Check sheet for the modelled part. Datum: model origin and axes. Units: mm. A direction names the side the tool comes from. Round coordinates to 2 decimals unless told otherwise and drop trailing zeros. Write each loop counter-clockwise with the first axis right and the second up, starting at its lowest first coordinate (ties: lowest second). Pieces come first, ordered by that corner, then holes.
Item 1: Release check for a two-part mould opening along Y. For faces 3 (the cylindrical face through (6.691, -12.864, -2.535)), 4 (the cylindrical face through (-17.34, -78.1, -0.07)), 5 (the flat face through (17, 1, 5)) record: +Y half, -Y half, draft (parallel to the pull), parting line (faces both ways), or undercut.
Item 2: Go/stop test with flat-tipped pins: pin 1 Ø5 at (y, z) = (-33, 1) entering from +X; pin 2 Ø1 at (x, z) = (-13, 3) entering from -Y; pin 3 Ø2 at (x, z) = (7, 0) entering from -Y. Record where each tip stops, or that it passes through.
Item 3: Material ranges on line 1 (Y direction, x = 0, z = -2.9); line 2 (Y direction, x = -6, z = -4); line 3 (Z direction, x = -16, y = -27.5), recorded low to high.
Item 4: Cross-section at D-D on x = 39.5. Enter the section's corners in (y, z), plus the area to 3 significant figures.
Item 5: Cross-section at A-A on y = 0. Enter the section's corners in (x, z).
Item 6: Cross-section at C-C on z = 2. Enter the section's corners in (x, y), plus the area to 3 significant figures.
Item 7: Tool access check on faces 1 (the flat face through (2, 12, -5)), 2 (the cylindrical face through (-58.23, 53.39, -2.54)). Record the directions out of +Z, -Z, +X, -X, +Y, -Y that give a thin tool (end or side, any length) a straight path to the whole face; none if there is none.
from build123d import *

# Parameters (mm, degrees)
SKETCH1_R           = 80
SKETCH1_R_2         = 12
BOSS_EXTRUDE1_DEPTH = 5
BOSS_EXTRUDE2_START = -10
SKETCH2_R           = 14.5
SKETCH2_R_2         = 12
BOSS_EXTRUDE2_DEPTH = 10
BOSS_EXTRUDE3_START = -10
SKETCH3_R           = 80
SKETCH3_R_2         = 79
BOSS_EXTRUDE3_DEPTH = 10


with BuildPart() as part:
    # Sketch1 → Boss-Extrude1 (new body)
    with BuildSketch(Plane.XY):
        Circle(SKETCH1_R)
        Circle(SKETCH1_R_2, mode=Mode.SUBTRACT)
    extrude(amount=BOSS_EXTRUDE1_DEPTH)

    # Sketch2 → Boss-Extrude2 (add)
    with BuildSketch(Plane.XY.offset(5).offset(BOSS_EXTRUDE2_START)):
        Circle(SKETCH2_R)
        Circle(SKETCH2_R_2, mode=Mode.SUBTRACT)
    extrude(amount=BOSS_EXTRUDE2_DEPTH)

    # Sketch3 → Boss-Extrude3 (add)
    with BuildSketch(Plane.XY.offset(5).offset(BOSS_EXTRUDE3_START)):
        Circle(SKETCH3_R)
        Circle(SKETCH3_R_2, mode=Mode.SUBTRACT)
    extrude(amount=BOSS_EXTRUDE3_DEPTH)


solid = part.part
Response values:
1. face 3: undercut
1. face 4: parting line
1. face 5: draft
2. pin 1: stops at x = 73.96
2. pin 2: stops at y = -79.02
2. pin 3: stops at y = -79.77
3. line 1: y = -80 to -79, -14.5 to -12, 12 to 14.5, 79 to 80
3. line 2: y = -79.77 to -78.77, -13.2 to -10.39, 10.39 to 13.2, 78.77 to 79.77
3. line 3: z = 0 to 5
4. outline: (-69.57, -5) - (-68.42, -5) - (-68.42, 0) - (68.42, 0) - (68.42, -5) - (69.57, -5) - (69.57, 5) - (-69.57, 5) - close
4. area: 707 mm2
5. outline: (-80, -5) - (-79, -5) - (-79, 0) - (-14.5, 0) - (-14.5, -5) - (-12, -5) - (-12, 5) - (-80, 5) - close; (12, -5) - (14.5, -5) - (14.5, 0) - (79, 0) - (79, -5) - (80, -5) - (80, 5) - (12, 5) - close
6. outline: circle Ø160 at (0, 0); hole circle Ø24 at (0, 0)
6. area: 19,700 mm2
7. face 1: -Z, +X, -X, +Y, -Y
7. face 2: -Z
